CAD build for the part. Positions are in the model's coordinates, mm. A direction names the side the tool comes from. Give positions to 0.01 mm unless a question says otherwise; leave off trailing zeros. Write each loop counter-clockwise with the first axis right and the second up, starting at its lowest first coordinate (ties: lowest second). Pieces come first, ordered by that corner, then holes. Notation, with made-up numbers: (-37.75, 42) - (-11.75, 42) arc R34 ccw to (-11.75, 72) - close; hole circle Ø2 at (59.25, 0.5). An arc over 180 degrees is marked (long way). Answer as a JSON object with one key per item and string values.
from build123d import *

# Parameters (mm, degrees)
F0_R      = 20
F1_DEPTH  = 6
F3_R      = 12
F4_DEPTH  = 4.25
F6_R      = 12.75
F7_DEPTH  = 5.5
F9_R      = 12
F10_DEPTH = 4.25
F12_R     = 20
F13_DEPTH = 6
F14_SIZE2 = 1.4
F14_SIZE  = 6
F15_SIZE2 = 6
F15_SIZE  = 1.4


with BuildPart() as f1:
    # F0 (on Top) → F1 (new body)
    with BuildSketch(Plane.XY):
        Circle(F0_R)
    extrude(amount=F1_DEPTH)

    # F3 (on offset) → F4 (join)
    with BuildSketch(Plane.XY.offset(6)):
        Circle(F3_R)
    extrude(amount=F4_DEPTH)

    # F6 (on offset) → F7 (join)
    with BuildSketch(Plane.XY.offset(10.25)):
        Circle(F6_R)
    extrude(amount=F7_DEPTH)

    # F9 (on offset) → F10 (join)
    with BuildSketch(Plane.XY.offset(15.75)):
        Circle(F9_R)
    extrude(amount=F10_DEPTH)

    # F12 (on offset) → F13 (join)
    with BuildSketch(Plane.XY.offset(20)):
        Circle(F12_R)
    extrude(amount=F13_DEPTH)

    # F14
    f14_edges = [f1.edges().sort_by_distance(p)[0] for p in [
        (-20, 0, 6),
    ]]
    f14_side = f1.faces().sort_by_distance((-19.434315, 0, 6))[0]
    chamfer(f14_edges, length=F14_SIZE, length2=F14_SIZE2, reference=f14_side)

    # F15
    f15_edges = [f1.edges().sort_by_distance(p)[0] for p in [
        (-20, 0, 20),
    ]]
    f15_side = f1.faces().sort_by_distance((-20, 0, 23))[0]
    chamfer(f15_edges, length=F15_SIZE, length2=F15_SIZE2, reference=f15_side)


solid = f1.part
(1) 3-axis set-ups, long thin cutter, end or side, ignore diameter. For faces 1 (the face through (-4.336, -19.524, 2.268)), 2 (the face through (-11.34, -8.7, 20.07)): which of +Z, -Z, +X, -X, +Y, -Y reach the whole face in a straight line?
Answer key:
{"face 1": "+Z, -Z", "face 2": "none"}
(2) Probe L1, parallel to Z at x = 12, y = 5; L2, parallel to Z at x = 11, y = 14.5; L3, parallel to Y at x = -9, z = 4.25. List the from-to ranges inside material, lowest first. Write a range as [from, to].
Answer key:
{"L1": "z = [0, 6], [20, 26]", "L2": "z = [0, 5.02], [20.98, 26]", "L3": "y = [-17.86, 17.86]"}
(3) Flat gauge pins, fed straight in: P1, Ø10, axis at y = 15.5, z = 3.5, coming from the -X side; P2, Ø1.5, axis at y = -1, z = 10.5, coming from the -X side; P3, Ø1, axis at x = 14.5, z = 5, coming from the -Y side. Where does each tip first touch, or does it go through?
Answer key:
{"P1": "stops at x = -17.02", "P2": "stops at x = -12.75", "P3": "stops at y = -14.08"}
(4) Saw through at A-A, the plane x = 0. Give the cut face in (y, z).
Answer key:
{"outline": "(-20, 0) - (20, 0) - (20, 4.6) - (14, 6) - (12, 6) - (12, 10.25) - (12.75, 10.25) - (12.75, 15.75) - (12, 15.75) - (12, 20) - (14, 20) - (20, 21.4) - (20, 26) - (-20, 26) - (-20, 21.4) - (-14, 20) - (-12, 20) - (-12, 15.75) - (-12.75, 15.75) - (-12.75, 10.25) - (-12, 10.25) - (-12, 6) - (-14, 6) - (-20, 4.6) - close"}
(5) Saw through at D-D, the plane z = 16.25. Give the cut face in (x, y).
Answer key:
{"outline": "circle Ø24 at (0, 0)"}
(6) Saw through at C-C, the plane z = 2.5. Give the cut face in (x, y).
Answer key:
{"outline": "circle Ø40 at (0, 0)"}
(7) Pull direction Z, two halves, no side cores. Call faces 3 (the face through (0, 0, 26)), 4 (the face through (0, 0, 0)), 5 (the face through (-3.116, -14.033, 5.912)), 6 (the face through (-4.336, -19.524, 23.668)): pulls with the +Z half, pulls with the -Z half, needs draft (parallel to the pull), parting line crosses it, or undercut.
Answer key:
{"face 3": "pulls with the +Z half", "face 4": "pulls with the -Z half", "face 5": "undercut", "face 6": "needs draft"}
